```python
from build123d import *

# Parameters (mm, degrees)
F0_W     = 200
F0_H     = 100
F1_DEPTH = 30
F2_R     = 20
F3_DEPTH = 60


with BuildPart() as f1:
    # F0 (on Front) → F1 (new body, symmetric)
    with BuildSketch(Plane.XZ):
        Rectangle(F0_W, F0_H)
    extrude(amount=F1_DEPTH, both=True)

    # F2 (on face) → F3 (cut, symmetric)
    with BuildSketch(Plane.XZ.offset(30)):
        Circle(F2_R)
    extrude(amount=F3_DEPTH, both=True, mode=Mode.SUBTRACT)


solid = f1.part
```
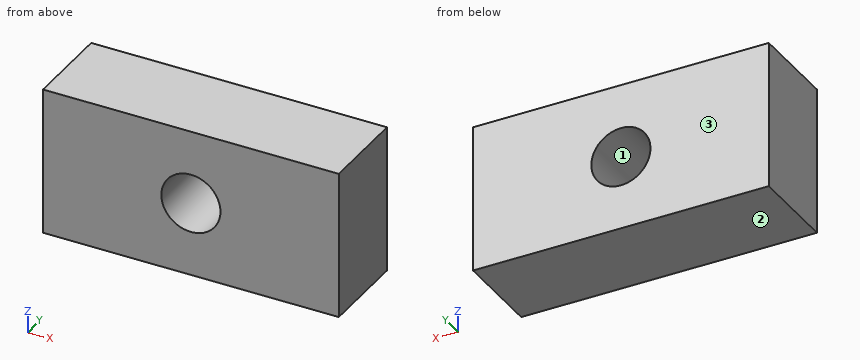
For this review, take the finished solid that the model builds, in its own axes (mm). Face numbers are marked on the shaded views. Give positions to 0.01 mm unless a question says otherwise; leave off trailing zeros. Order: outer loops, then holes, each group sorted by start corner. A loop starts at its lowest first (then second) coordinate and runs counter-clockwise, first axis right, second up.
1) Wall thickness on line 1 (Z direction, x = 0, y = 11); line 2 (X direction, y = -2.5, z = -5); line 3 (X direction, y = 16, z = 17.5): over which ranges is each line inside the solid? List them lowest first.
2) The part is to be moulded in two halves that separate along Z. For the marked faces 1, 2 and 3, say which applies: released by +Z, released by -Z, zero draft, split by the parting line, or undercut.
3) Take a section at C-C (y = -9.5). Give the boundary of the cut face in (x, z), then the cut area to 3 significant figures.
4) Take a section at A-A (x = 0). Give the boundary of the cut face in (y, z).
5) Take a section at B-B (z = 0). Give the boundary of the cut face in (x, y).
Derived:
1. line 1: z = -50 to -20, 20 to 50
1. line 2: x = -100 to -19.36, 19.36 to 100
1. line 3: x = -100 to -9.68, 9.68 to 100
2. face 1: undercut
2. face 2: released by -Z
2. face 3: zero draft
3. outline: (-100, -50) - (100, -50) - (100, 50) - (-100, 50) - close; hole circle Ø40 at (0, 0)
3. area: 18,700 mm2
4. outline: (-30, -50) - (30, -50) - (30, -20) - (-30, -20) - close; (-30, 20) - (30, 20) - (30, 50) - (-30, 50) - close
5. outline: (-100, -30) - (-20, -30) - (-20, 30) - (-100, 30) - close; (20, -30) - (100, -30) - (100, 30) - (20, 30) - close
